The figure shows three views and two pictorial views of one solid part (mm, origin at its lowest corner). Answer the questions. A direction names the side the tool comes from. Give positions to 0.01 mm unless a question says otherwise; leave off trailing zeros. Write each loop counter-clockwise with the first axis right and the second up, starting at its lowest first coordinate (ties: lowest second). Pieces come first, ordered by that corner, then holes. Notation, with made-up numbers: (9, 12) -> (20, 12) arc R35 cw to (20, 46) -> close; hole circle Ø4 at (33.5, 59.25). An arc over 180 degrees is marked (long way). Use a Markdown table: item, result.
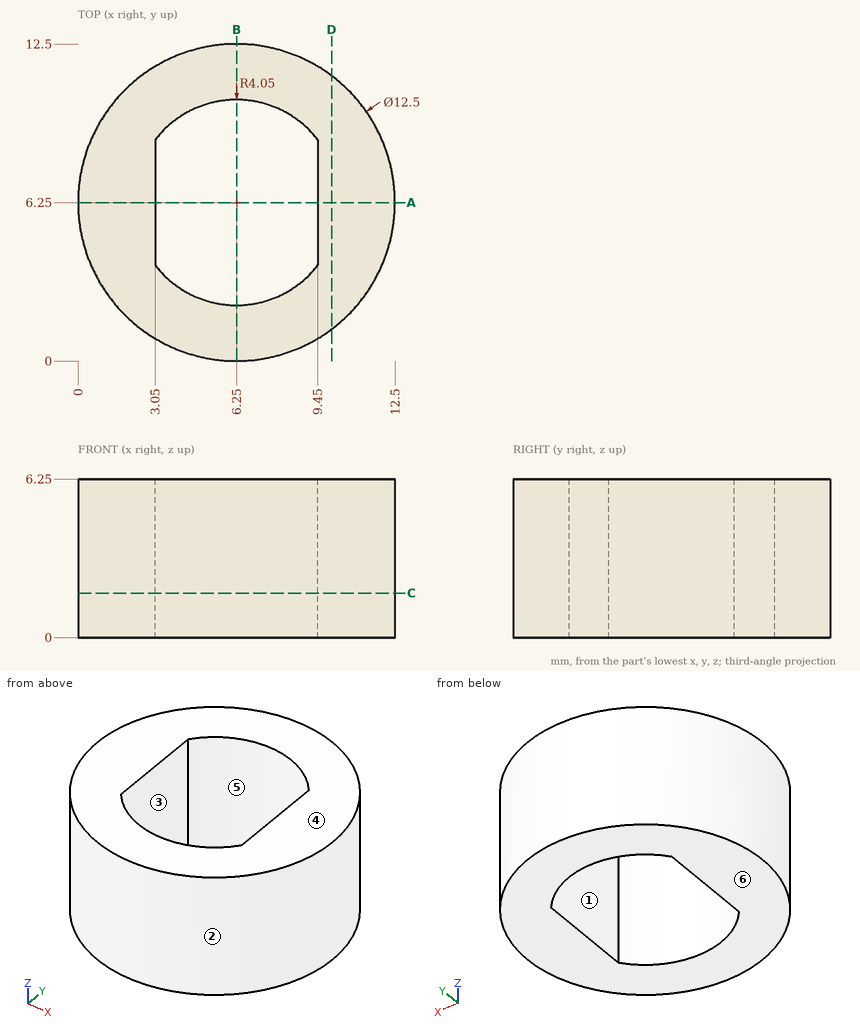
Item 1: A cutting plane is placed at A-A (y = 6.25). Give the vertices of the cut face in (x, z), then the cut area to 3 significant figures.
Return value:
| item | result |
|---|---|
| outline | (0, 0) -> (3.05, 0) -> (3.05, 6.25) -> (0, 6.25) -> close; (9.45, 0) -> (12.5, 0) -> (12.5, 6.25) -> (9.45, 6.25) -> close |
| area | 38.1 mm^2 |
Item 2: A cutting plane is placed at B-B (x = 6.25). Give the vertices of the cut face in (y, z).
Return value:
| item | result |
|---|---|
| outline | (0, 0) -> (2.2, 0) -> (2.2, 6.25) -> (0, 6.25) -> close; (10.3, 0) -> (12.5, 0) -> (12.5, 6.25) -> (10.3, 6.25) -> close |
Item 3: A cutting plane is placed at C-C (z = 1.75). Give the vertices of the cut face in (x, y), then the cut area to 3 significant figures.
Return value:
| item | result |
|---|---|
| outline | circle Ø12.5 at (6.25, 6.25); hole (3.05, 3.77) arc R4.05 ccw to (9.45, 3.77) -> (9.45, 8.73) arc R4.05 ccw to (3.05, 8.73) -> close |
| area | 76.9 mm^2 |
Item 4: A cutting plane is placed at D-D (x = 10). Give the vertices of the cut face in (y, z), then the cut area to 3 significant figures.
Return value:
| item | result |
|---|---|
| outline | (1.25, 0) -> (11.25, 0) -> (11.25, 6.25) -> (1.25, 6.25) -> close |
| area | 62.5 mm^2 |
Item 5: For a pull along X with two mould halves and no side action, classify the marked faces 1, 2, 3 and 4 as +X half, -X half, draft (parallel to the pull), parting line (faces both ways), or undercut.
Return value:
| item | result |
|---|---|
| face 1 | undercut |
| face 2 | parting line |
| face 3 | undercut |
| face 4 | draft |
Item 6: A tool of negligible diameter and unlimited length cuts with its end or side. For the marked faces 5 and 6, from which of +Z, -Z, +X, -X, +Y, -Y can it reach the whole face along a straight path? Write none if from no direction.
Return value:
| item | result |
|---|---|
| face 5 | +Z, -Z |
| face 6 | -Z, +X, -X, +Y, -Y |
Item 7: Straight lines are drawn through the part: line 1 along Y through (x, z) = (6.75, 3.5); line 2 along X through (y, z) = (9.25, 4); line 3 along X through (y, z) = (3, 4.75). For each, find the intervals that lie inside material, in ascending order. Write a range as [from, to].
Return value:
| item | result |
|---|---|
| line 1 | [0.02, 2.23], [10.27, 12.48] |
| line 2 | [0.77, 3.53], [8.97, 11.73] |
| line 3 | [0.91, 3.83], [8.67, 11.59] |
Item 8: Each of these flat-tipped pins is pushed along its axis until it touches: P1, Ø1.5, axis at x = 4.5, z = 1, coming from the +Y side; P2, Ø2, axis at x = 2.5, z = 4.5, coming from the +Y side. Where does it stop, or does it pass through?
Return value:
| item | result |
|---|---|
| P1 | y = 12.42 |
| P2 | y = 11.86 |
